Check sheet for the modelled part. Datum: model origin and axes. Units: mm. A direction names the side the tool comes from. Give positions to 0.01 mm unless a question says otherwise; leave off trailing zeros. Loops run counter-clockwise (first coordinate to the right, second up) from the corner with the lowest first, then second, coordinate; pieces in that order, holes last. Notation, with made-up numbers: M -38.5,61 L -27.5,61 A26 ccw -27.5,89 Z; hole C -28.5,15.25 d1. An arc over 180 degrees is marked long. Use one line per item in the form item = value.
from build123d import *

# Parameters (mm, degrees)
PAD_DEPTH       = 15
SKETCH001_R     = 2.2
POCKET_DEPTH    = 15.914024
POCKET001_DEPTH = 2.5


with BuildPart() as part:
    # Sketch → Pad (new body)
    with BuildSketch(Plane.XY):
        with BuildLine():
            Line((-12.7, -13.086976), (-8.7, -13.086976))
            Line((-8.7, -13.086976), (-8.7, -17.086976))
            Line((-8.7, -17.086976), (-16.7, -17.086976))
            Line((-16.7, -17.086976), (-16.7, 2.913024))
            ThreePointArc((-3.7, 15.913024), (-12.892388, 12.105412), (-16.7, 2.913024))
            Line((-3.7, 15.913024), (3.7, 15.913024))
            ThreePointArc((16.7, 2.913024), (12.892388, 12.105412), (3.7, 15.913024))
            Line((16.7, 2.913024), (16.7, -17.086976))
            Line((16.7, -17.086976), (8.7, -17.086976))
            Line((8.7, -17.086976), (8.7, -13.086976))
            Line((8.7, -13.086976), (12.7, -13.086976))
            Line((12.7, -13.086976), (12.7, 2.913024))
            ThreePointArc((12.7, 2.913024), (10.063961, 9.276985), (3.7, 11.913024))
            Line((3.7, 11.913024), (-3.7, 11.913024))
            ThreePointArc((-3.7, 11.913024), (-10.063961, 9.276985), (-12.7, 2.913024))
            Line((-12.7, 2.913024), (-12.7, -13.086976))
        make_face()
    extrude(amount=PAD_DEPTH)

    # Sketch001 → Pocket (cut, through all)
    with BuildSketch(Plane.XZ):
        with Locations((0, 7.5)):
            Circle(SKETCH001_R)
    extrude(amount=-POCKET_DEPTH, mode=Mode.SUBTRACT)

    # Sketch002 (on Face11 of Pocket) → Pocket001 (cut, symmetric)
    with BuildSketch(Plane.XZ.offset(-11.913024)):
        Polygon((2.136196, 11.2), (-2.136196, 11.2), (-4.272392, 7.5), (-2.136196, 3.8), (2.136196, 3.8), (4.272392, 7.5), align=None)
    extrude(amount=POCKET001_DEPTH, both=True, mode=Mode.SUBTRACT)


solid = part.part
1) Section check C-C (z = 14). Record the cut outline in (x, y), then the cut area to 3 significant figures.
Evaluation:
outline = M -16.7,-17.09 L -8.7,-17.09 L -8.7,-13.09 L -12.7,-13.09 L -12.7,2.91 A9 cw -3.7,11.91 L 3.7,11.91 A9 cw 12.7,2.91 L 12.7,-13.09 L 8.7,-13.09 L 8.7,-17.09 L 16.7,-17.09 L 16.7,2.91 A13 ccw 3.7,15.91 L -3.7,15.91 A13 ccw -16.7,2.91 Z
area = 360 mm^2
2) Scan lines: line 1 (X direction, y = -0.5, z = 5.5); line 2 (X direction, y = -15, z = 12); line 3 (Z direction, x = 0, y = 14.95). Record each from-to range of solid material in increasing order.
Evaluation:
line_1 = -16.7 to -12.7, 12.7 to 16.7
line_2 = -16.7 to -8.7, 8.7 to 16.7
line_3 = 0 to 5.3, 9.7 to 15
3) Set-up check for faces 1 (the face through (11, -13.087, 7)), 2 (the face through (-8.7, -15, 7)), 3 (the face through (3.189, 13.136, 5.624)): record each of +Z, -Z, +X, -X, +Y, -Y from which the full face is reachable in a straight line by a thin tool's end or side.
Evaluation:
face_1 = +Z, -Z
face_2 = +Z, -Z, -Y
face_3 = -Y
4) Release check for a two-part mould opening along X. For faces 4 (the face through (2, 14.413, 6)), 5 (the face through (-1, 13, 15)), 6 (the face through (12.993, 12.004, 7.395)) record: pulls with the +X half, pulls with the -X half, needs draft (parallel to the pull), parting line crosses it, or undercut.
Evaluation:
face_4 = undercut
face_5 = needs draft
face_6 = pulls with the +X half
5) Section check A-A (y = -6). Record the cut outline in (x, z).
Evaluation:
outline = M -16.7,0 L -12.7,0 L -12.7,15 L -16.7,15 Z; M 12.7,0 L 16.7,0 L 16.7,15 L 12.7,15 Z
6) Section check D-D (z = 6). Record the cut outline in (x, y).
Evaluation:
outline = M -16.7,-17.09 L -8.7,-17.09 L -8.7,-13.09 L -12.7,-13.09 L -12.7,2.91 A9 cw -3.7,11.91 L -3.41,11.91 L -3.41,14.41 L -1.61,14.41 L -1.61,15.91 L -3.7,15.91 A13 ccw -16.7,2.91 Z; M 1.61,14.41 L 3.41,14.41 L 3.41,11.91 L 3.7,11.91 A9 cw 12.7,2.91 L 12.7,-13.09 L 8.7,-13.09 L 8.7,-17.09 L 16.7,-17.09 L 16.7,2.91 A13 ccw 3.7,15.91 L 1.61,15.91 Z
7) Section check B-B (x = 0). Record the cut outline in (y, z), then the cut area to 3 significant figures.
Evaluation:
outline = M 11.91,0 L 15.91,0 L 15.91,5.3 L 14.41,5.3 L 14.41,3.8 L 11.91,3.8 Z; M 11.91,11.2 L 14.41,11.2 L 14.41,9.7 L 15.91,9.7 L 15.91,15 L 11.91,15 Z
area = 34.9 mm^2
8) Depth check by flat-ended pin: pin 1 Ø3.5 at (x, z) = (1, 4.5) entering from -Y; pin 2 Ø8 at (x, z) = (-4.5, 6.5) entering from -Y; pin 3 Ø6 at (x, z) = (2, 8.5) entering from -Y. Enter the tip coordinate at first touch or a pass-through.
Evaluation:
pin_1 = 11.91
pin_2 = 10.53
pin_3 = 11.82
